Autodesk Inventor part; units mm, degrees
ref_plane "YZ Plane" through (0, 0, 0) normal (1, 0, 0) x (0, 1, 0)
ref_plane "XZ Plane" through (0, 0, 0) normal (0, 1, 0) x (-1, 0, 0)
ref_plane "XY Plane" through (0, 0, 0) normal (0, 0, 1) x (1, 0, 0)
sketch "Sketch1" plane through (0, 0, 0) normal (0, 1, 0) x (-1, 0, 0)
  line L0 (25.4, 25.4) -> (-25.4, 25.4)
  line L1 (-25.4, 25.4) -> (-25.4, -22.225)
  line L2 (-25.4, -22.225) -> (25.4, -22.225)
  line L3 (25.4, -22.225) -> (25.4, 25.4)
  point P0 (0, 0)
  dimension "d0" = 50.8
  dimension "d1" = 47.625
  dimension "d2" = 25.4
  dimension "d3" = 25.4
extrude "Extrusion1" add sketch "Sketch1" along normal blind 3.175
sketch "Sketch4" plane through (-25.4, 0, -19.05) normal (0, 0, -1) x (-1, 0, 0)
  line L0 (-50.8, 0) -> (0, 0)
  line L1 (0, 0) -> (0, 25.4)
  line L2 (0, 25.4) -> (-50.8, 25.4)
  line L3 (-50.8, 25.4) -> (-50.8, 0)
edge flange "Flange1" height 25.4 angle 90 thickness 3.175 bend radius 3.175 thickness toward (0, 0, -1) relief tear relief width 3.175 relief depth 1.5875 edges at (0, 3.175, -22.225) wall of the first edge with corners at (25.4, 0, -19.05) (-25.4, 0, -19.05) (-25.4, 25.4, -19.05) (25.4, 25.4, -19.05)
bend "Bend1"
corner "Corner1"
sketch "Sketch5" plane through (0, 3.175, 0) normal (0, 1, 0) x (1, 0, 0)
  line L0 (-25.4, -25.4) -> (25.4, -25.4)
  line L1 (-25.4, 15.875) -> (-25.4, -25.4)
  point P0 (0, 0)
  point P1 (-12.7, -16.256)
  point P2 (12.7, -16.256)
  dimension "d23" = 9.144
  dimension "d24" = 9.144
  dimension "d25" = 25.4
  dimension "d26" = 12.7
hole "Hole1" at (-12.7, 3.175, 16.256) at (12.7, 3.175, 16.256) direction (0, -1, 0) diameter 6.35 end through all
sketch "Sketch6" plane through (25.4, 25.4, -22.225) normal (0, 0, -1) x (-1, 0, 0)
  line L0 (0, 0) -> (50.8, 0)
  line L1 (50.8, 0) -> (50.8, -19.05)
  point P0 (25.4, -25.4)
  point P1 (25.4, -12.7)
  dimension "d34" = 12.7
  dimension "d35" = 25.4
hole "Hole2" at (0, 12.7, -22.225) direction (0, 0, 1) diameter 6.35 end through all
equation "\"d32\" = Thickness"
equation "\"d41\" = Thickness"
equation "\"d13\" = BendReliefWidth"
equation "\"d14\" = BendReliefDepth"
equation "\"d15\" = MinimumRemnant"
equation "\"d16\" = BendRadius"
equation "\"d19\" = BendRadius"
equation "\"d20\" = CornerReliefSize"
equation "\"d21\" = GapSize"
equation "\"d22\" = JacobiRadiusSize"
equation "\"BendRadius\" = Thickness"
equation "\"BendReliefWidth\" = Thickness"
equation "\"BendReliefDepth\" = 0.5 * Thickness"
equation "\"CornerReliefSize\" = 4 * Thickness"
equation "\"MinimumRemnant\" = 2 * Thickness"
equation "\"TransitionRadius\" = BendRadius"
equation "\"JacobiRadiusSize\" = BendRadius"
equation "\"GapSize\" = Thickness"
properties part number "Sheet for"
Check sheet for the modelled part. Datum: model origin and axes. Units: mm. A direction names the side the tool comes from. Give positions to 0.01 mm unless a question says otherwise; leave off trailing zeros. Write each loop counter-clockwise with the first axis right and the second up, starting at its lowest first coordinate (ties: lowest second). Pieces come first, ordered by that corner, then holes. Notation, with made-up numbers: (25, 6) -> (57, 6) arc R30 cw to (57, 33) -> close; hole circle Ø1 at (40.5, 12). An arc over 180 degrees is marked (long way). One line per item, written item: value. Start each with the question number.
Item 1: Section check D-D on z = 6. Record the cut outline in (x, y) (3 decimals).
Item 2: Tool access check on faces 1 (the flat face through (0, 3.175, 5)), 2 (the cylindrical face through (-0.14, 9.53, -20.62)). Record the directions out of +Z, -Z, +X, -X, +Y, -Y that give a thin tool (end or side, any length) a straight path to the whole face; none if there is none.
Item 3: Material ranges on probe 1 along X at (y, z) = (12.7, -19.95) (3 decimals); probe 2 along Y at (x, z) = (9, 13) (3 decimals); probe 3 along Z at (x, y) = (14.5, 20) (3 decimals), recorded low to high. Write a range as from..to.
Item 4: Section check C-C on x = 21. Record the cut outline in (y, z) (3 decimals), then the cut area to 3 significant figures.
Item 5: Draft check along Z on faces 3 (the cylindrical face through (-11.484, 1.565, 19.189)), 4 (the flat face through (25.4, 2, -7)), 5 (the flat face through (0, 18, -19.05)), 6 (the cylindrical face through (13.916, 1.565, 19.189)). Enter one of: +Z half, -Z half, draft (parallel to the pull), parting line (faces both ways), or undercut.
Item 6: Gauge pin test, flat ends, axial feed: pin 1 (5.5 mm diameter, centred on x = -12.7, z = 16.256, fed in from +Y); pin 2 (4 mm diameter, centred on x = 9, y = 17, fed in from +Z). Record the tip position at first contact, or that the pin passes through.
Item 7: Section check A-A on x = -12.7. Record the cut outline in (y, z) (3 decimals).
Item 8: Section check B-B on y = 12.7. Record the cut outline in (x, z) (3 decimals).
Results list:
1. outline: (-25.4, 0) -> (25.4, 0) -> (25.4, 3.175) -> (-25.4, 3.175) -> close
2. face 1: +Z, +X, -X, +Y
2. face 2: +Z, -Z
3. probe 1: -25.4..-3.175, 3.175..25.4
3. probe 2: 0..3.175
3. probe 3: -22.225..-19.05
4. outline: (0, -15.875) arc R6.35 ccw to (6.35, -22.225) -> (25.4, -22.225) -> (25.4, -19.05) -> (6.35, -19.05) arc R3.175 cw to (3.175, -15.875) -> (3.175, 25.4) -> (0, 25.4) -> close
4. area: 215 mm²
5. face 3: undercut
5. face 4: draft
5. face 5: +Z half
5. face 6: undercut
6. pin 1: through
6. pin 2: z = -19.05
7. outline: (0, -15.875) arc R6.35 ccw to (6.35, -22.225) -> (25.4, -22.225) -> (25.4, -19.05) -> (6.35, -19.05) arc R3.175 cw to (3.175, -15.875) -> (3.175, 13.081) -> (0, 13.081) -> close; (0, 19.431) -> (3.175, 19.431) -> (3.175, 25.4) -> (0, 25.4) -> close
8. outline: (-25.4, -22.225) -> (-3.175, -22.225) -> (-3.175, -19.05) -> (-25.4, -19.05) -> close; (3.175, -22.225) -> (25.4, -22.225) -> (25.4, -19.05) -> (3.175, -19.05) -> close
